from build123d import *

# Parameters (mm, degrees)
F0_W     = 25.4
F0_H     = 76.2
F0_W_2   = 20.32
F0_H_2   = 7.62
F1_ANGLE = 20
F2_W     = 2.54
F2_H     = 76.2
F2_W_2   = 2.7023823932
F2_H_2   = 76.3387009501
F3_DEPTH = 5.08
F4_W     = 2.54
F4_H     = 11.1115600293
F4_H_2   = 8.0921141291
F4_H_3   = 5.7973351781
F4_H_4   = 3.5076183132
F4_H_5   = 2.4190474503
F4_H_6   = 1.4033722508
F5_DEPTH = 25.401


with BuildPart() as f1:
    # F0 (on Top) → F1 (revolve)
    with BuildSketch(Plane.XY):
        with Locations((0.1395599202, 38.1)):
            Rectangle(F0_W, F0_H)
        with Locations((0.1395599202, 19.05)):
            Rectangle(F0_W_2, F0_H_2, mode=Mode.SUBTRACT)
        with Locations((0.1395599202, 29.21)):
            Rectangle(F0_W_2, F0_H_2, mode=Mode.SUBTRACT)
        with Locations((0.1395599202, 39.37)):
            Rectangle(F0_W_2, F0_H_2, mode=Mode.SUBTRACT)
        with Locations((0.1395599202, 49.53)):
            Rectangle(F0_W_2, F0_H_2, mode=Mode.SUBTRACT)
        with Locations((0.1395599202, 59.69)):
            Rectangle(F0_W_2, F0_H_2, mode=Mode.SUBTRACT)
        with Locations((0.1395599202, 69.85)):
            Rectangle(F0_W_2, F0_H_2, mode=Mode.SUBTRACT)
    revolve(axis=Axis((0.1395599202, 0, 0), (1, 0, 0)), revolution_arc=F1_ANGLE)

    # F2 (on face) → F3 (join)
    with BuildSketch(Plane(origin=(0, 0, 0), x_dir=(1, 0, 0), z_dir=(0, -0.3420201433, 0.9396926208))):
        with Locations((-11.2904400798, 38.1)):
            Rectangle(F2_W, F2_H)
        with Locations((11.6798062809, 38.1693504751)):
            Rectangle(F2_W_2, F2_H_2)
    extrude(amount=F3_DEPTH)

    # F4 (on face) → F5 (cut, through all)
    with BuildSketch(Plane.YZ.offset(12.8395599202)):
        with Locations((69.3939362815, 9.8744578206)):
            Rectangle(F4_W, F4_H)
        with Locations((58.834955257, 8.3647348704)):
            Rectangle(F4_W, F4_H_2)
        with Locations((48.8164393489, 7.3381234978)):
            Rectangle(F4_W, F4_H_3)
        with Locations((39.3121916656, 5.9616579595)):
            Rectangle(F4_W, F4_H_4)
        with Locations((30.3617200801, 5.0545152959)):
            Rectangle(F4_W, F4_H_5)
        with Locations((20.0811068022, 3.1433054453)):
            Rectangle(F4_W, F4_H_6)
    extrude(amount=-F5_DEPTH, mode=Mode.SUBTRACT)


solid = f1.part
Source: CAD feature listing. Evaluate the final solid. Frame: model axes, mm. A direction names the side the tool comes from. Give positions to 0.01 mm unless a question says otherwise; leave off trailing zeros. Write each loop counter-clockwise with the first axis right and the second up, starting at its lowest first coordinate (ties: lowest second). Pieces come first, ordered by that corner, then holes. Notation, with made-up numbers: M 50,23.25 L 92,23.25 A12 ccw 92,38.25 Z; hole C -12,-30 d11. An arc over 180 degrees is marked long. Return JSON: item names as keys, results as strings. Group by question number.
1) Cut plane D-D, the plane y = 11. Output: boundary loops of the cut face in (x, z).
2) Cut plane C-C, the plane z = 13.5. Give the number of separate pieces and of enclosed holes in the cut face, plus the area to 3 significant figures.
3) Cut plane A-A, the plane x = 9.5. Output: boundary loops of the cut face in (y, z), plus the area to 3 significant figures.
4) Material intervals for line 1 along X through (y, z) = (35.5, 11); line 2 along Y through (x, z) = (2.25, 17); line 3 along Y through (x, z) = (-7.25, 18), sorted ascending. Write a range as [from, to].
5) Pin query (flat end, axial travel): P1, Ø2, axis at x = -11, z = 5.5, coming from the +Y side; P2, Ø0.8, axis at x = -11, y = 69, coming from the +Z side; P3, Ø0.8, axis at x = -11, y = 30, coming from the +Z side; P4, Ø2, axis at x = 10.5, y = 23.5, coming from the -Z side. Return the tip coordinate at first contact, or that it passes through.
6) Pull-direction query (X, two-part tool) for faces 1 (the face through (-11, 30, 3.845)), 2 (the face through (10.3, 28.5, 5.7)); classes: pulls with the +X half, pulls with the -X half, needs draft (parallel to the pull), parting line crosses it, or undercut.
7) Set-up query: faces 3 (the face through (0.282, 42.542, 7.394)), 4 (the face through (12, 40.582, 6)), 5 (the face through (0.282, 25.025, 4.35)). Return all of +Z, -Z, +X, -X, +Y, -Y with unobstructed straight access to the full face (end or side cutting, diameter ignored); none if empty.
Recorded:
{
 "1": {"outline": "M -12.56,0 L 12.84,0 L 12.84,4 L 13.03,4 L 13.03,9.41 L 10.33,9.41 L 10.33,4 L -10.02,4 L -10.02,9.41 L -12.56,9.41 Z"},
 "2": {"separate pieces": "2", "enclosed holes": "2", "area": "470 mm²"},
 "3": {"outline": "M 0,0 L 15.24,0 A15.24 ccw 14.32,5.21 Z; M 21.48,7.82 A22.86 cw 22.86,0 L 25.4,0 A25.4 ccw 23.87,8.69 Z; M 31.03,11.29 A33.02 cw 33.02,0 L 35.56,0 A35.56 ccw 33.42,12.16 Z; M 40.58,14.77 A43.18 cw 43.18,0 L 45.72,0 A45.72 ccw 42.96,15.64 Z; M 50.12,18.24 A53.34 cw 53.34,0 L 55.88,0 A55.88 ccw 52.51,19.11 Z; M 59.67,21.72 A63.5 cw 63.5,0 L 66.04,0 A66.04 ccw 62.06,22.59 Z; M 69.22,25.19 A73.66 cw 73.66,0 L 76.2,0 A76.2 ccw 71.6,26.06 Z", "area": "304 mm²"},
 "4": {"line 1": "x = [-12.56, -10.02], [10.3, 12.84]", "line 2": "y = [50.56, 53.23], [61.18, 63.81], [71.67, 74.28]", "line 3": "y = [50.21, 52.9], [60.9, 63.54], [71.43, 74.04]"},
 "5": {"P1": "stops at y = 76.07", "P2": "stops at z = 30.67", "P3": "stops at z = 16.47", "P4": "stops at z = 0"},
 "6": {"face 1": "needs draft", "face 2": "undercut"},
 "7": {"face 3": "-Z", "face 4": "+X, -X", "face 5": "+Z"}
}
